Check sheet for the modelled part. Datum: model origin and axes. Units: mm. Round coordinates to 2 decimals unless told otherwise and drop trailing zeros. Write each loop counter-clockwise with the first axis right and the second up, starting at its lowest first coordinate (ties: lowest second). Pieces come first, ordered by that corner, then holes. Notation, with made-up numbers: M -5.5,66.5 L 51.5,66.5 A11 ccw 51.5,76.5 Z; hole C -33.5,-16 d9. An arc over 180 degrees is marked long. One line per item, written item: value.
from build123d import *

# Parameters (mm, degrees)
SKETCH3_R = 0.1


with BuildPart() as part:
    # Sketch1 → Revolve1 (revolve)
    with BuildSketch(Plane.XY, mode=Mode.PRIVATE) as revolve1_sk:
        with BuildLine():
            Line((2.5, 0), (2.5, 0.5))
            ThreePointArc((2.5, 0.5), (2.353553391, 0.853553391), (2, 1))
            Line((2, 1), (-2, 1))
            ThreePointArc((-2, 1), (-2.353553391, 0.853553391), (-2.5, 0.5))
            Line((-2.5, 0.5), (-2.5, 0))
            Line((-2.5, 0), (2.5, 0))
        make_face()
    revolve(revolve1_sk.sketch.rotate(Axis((15.850565012, 0, 0), (-1, 0, 0)), 90), axis=Axis((15.850565012, 0, 0), (-1, 0, 0)))

    # Sweep1: sweep along a path in Sketch2
    with BuildLine(Plane.XY) as sweep1_path:
        Line((2.5, 0), (4, 0))
        ThreePointArc((4, 0), (4.707106781, -0.292893219), (5, -1))
        Line((5, -1), (5, -20))
    # Sketch3 → Sweep1 (sweep)
    with BuildSketch(Plane(origin=(2.5, 0, 0), x_dir=(0, 0, -1), z_dir=(1, 0, 0))):
        Circle(SKETCH3_R)
    sweep1 = sweep(path=sweep1_path.line)

    # Mirror1: Sweep1 across plane
    add(sweep1.mirror(Plane(origin=(0, 0, 0), x_dir=(0, 0, 1), z_dir=(1, 0, 0))))


solid = part.part
Q1. Depth check by flat-ended pin: P1, Ø1, axis at x = -4, y = -9.5, coming from the -Z side; P2, Ø0.8, axis at y = 0, z = 0, coming from the -X side. Enter the tip coordinate at first touch or a pass-through.
Completed:
P1: through
P2: x = -4.92
Q2. Scan lines: line 1 (Y direction, x = 1.25, z = -0.5); line 2 (Y direction, x = 1.75, z = -0.55); line 3 (X direction, y = -0.5, z = 0.6). Record each from-to range of solid material in increasing order. Write a range as [from, to].
Completed:
line 1: [-0.87, 0.87]
line 2: [-0.84, 0.84]
line 3: [-2.41, 2.41]
Q3. Sectioned sample at B-B on x = 2.75. Enter the section's corners in (y, z).
Completed:
outline: C 0,0 d0.2
Q4. Sectioned sample at A-A on y = -2.25. Enter the section's corners in (x, z), and give its area (3 significant figures).
Completed:
outline: C -5,0 d0.2; C 5,0 d0.2
area: 0.0628 mm^2
Q5. Sectioned sample at C-C on x = 1.25. Enter the section's corners in (y, z).
Completed:
outline: C 0,0 d2
